from build123d import *

# Parameters (mm, degrees)
SKETCH1_R           = 9.525
BOSS_EXTRUDE1_DEPTH = 10.922
SKETCH2_R           = 4.7625
BOSS_EXTRUDE2_DEPTH = 9.525
BOSS_EXTRUDE3_DEPTH = 12.7


with BuildPart() as part:
    # Sketch1 → Boss-Extrude1 (new body)
    with BuildSketch(Plane(origin=(0, 0, 0), x_dir=(1, 0, 0), z_dir=(0, 1, 0))):
        Circle(SKETCH1_R)
    extrude(amount=BOSS_EXTRUDE1_DEPTH)

    # Sketch2 → Boss-Extrude2 (add)
    with BuildSketch(Plane(origin=(0, 10.922, 0), x_dir=(1, 0, 0), z_dir=(0, 1, 0))):
        Circle(SKETCH2_R)
    extrude(amount=BOSS_EXTRUDE2_DEPTH)

    # Sketch3 → Boss-Extrude3 (add)
    with BuildSketch(Plane(origin=(0, 20.447, 0), x_dir=(1, 0, 0), z_dir=(0, 1, 0))):
        with BuildLine():
            Line((-2.20336765, 2.286), (2.20336765, 2.286))
            ThreePointArc((2.20336765, 2.286), (0, -3.175), (-2.20336765, 2.286))
        make_face()
    extrude(amount=BOSS_EXTRUDE3_DEPTH)


solid = part.part
Geometry: final body of the model. Coordinates: model frame, mm. A direction names the side the tool comes from. Give positions to 0.01 mm unless a question says otherwise; leave off trailing zeros. Write each loop counter-clockwise with the first axis right and the second up, starting at its lowest first coordinate (ties: lowest second). Pieces come first, ordered by that corner, then holes. Notation, with made-up numbers: (7.5, 36.5) -> (38.5, 36.5) arc R36 ccw to (38.5, 71.5) -> close; hole circle Ø3 at (84, 21.25). An arc over 180 degrees is marked (long way). Answer in a Markdown table with one row per item.
(1) Ray query, line 1 along Y through (x, z) = (4.5, 2.75); line 2 along Y through (x, z) = (3, 2.5); line 3 along X through (y, z) = (31, 0.75). Return the intervals inside material, ascending. Write a range as [from, to].
Answers below:
| item | result |
|---|---|
| line 1 | [0, 10.92] |
| line 2 | [0, 20.45] |
| line 3 | [-3.09, 3.09] |
(2) Section query D-D on y = 4.5. Return loops of the section in (x, z) (3 decimals), then the cut area to 3 significant figures.
Answers below:
| item | result |
|---|---|
| outline | circle Ø19.05 at (0, 0) |
| area | 285 mm^2 |
(3) Pin query (flat end, axial travel): pin 1 (2 mm diameter, centred on y = 7, z = -7.5, fed in from -X); pin 2 (1.5 mm diameter, centred on x = -1, y = 19.5, fed in from -Z); pin 3 (3.5 mm diameter, centred on x = -0.5, y = 26.5, fed in from -Z). Return the tip coordinate at first contact, or that it passes through.
Answers below:
| item | result |
|---|---|
| pin 1 | x = -6.96 |
| pin 2 | z = -4.76 |
| pin 3 | z = -2.29 |
(4) Section query C-C on y = 30. Return loops of the section in (x, z) (3 decimals).
Answers below:
| item | result |
|---|---|
| outline | (-2.203, -2.286) -> (2.203, -2.286) arc R3.175 ccw (long way) to start |
(5) Section query B-B on x = 0. Return loops of the section in (y, z) (1 decimal), then the cut area to 3 significant figures.
Answers below:
| item | result |
|---|---|
| outline | (0, -9.5) -> (10.9, -9.5) -> (10.9, -4.8) -> (20.4, -4.8) -> (20.4, -2.3) -> (33.1, -2.3) -> (33.1, 3.2) -> (20.4, 3.2) -> (20.4, 4.8) -> (10.9, 4.8) -> (10.9, 9.5) -> (0, 9.5) -> close |
| area | 368 mm^2 |
(6) Set-up query: faces 1 (the flat face through (-4.4, 10.922, -2.3)), 2 (the flat face through (0, 27, -2.286)), 3 (the cylindrical face through (-7.559, 5.385, 5.796)). Return all of +Z, -Z, +X, -X, +Y, -Y with unobstructed straight access to the full face (end or side cutting, diameter ignored); none if empty.
Answers below:
| item | result |
|---|---|
| face 1 | +Y |
| face 2 | -Z, +X, -X, +Y |
| face 3 | +Y, -Y |
(7) Section query A-A on z = 0. Return loops of the section in (x, y) (1 decimal), then the cut area to 3 significant figures.
Answers below:
| item | result |
|---|---|
| outline | (-9.5, 0) -> (9.5, 0) -> (9.5, 10.9) -> (4.8, 10.9) -> (4.8, 20.4) -> (3.2, 20.4) -> (3.2, 33.1) -> (-3.2, 33.1) -> (-3.2, 20.4) -> (-4.8, 20.4) -> (-4.8, 10.9) -> (-9.5, 10.9) -> close |
| area | 379 mm^2 |
